from build123d import *

# Parameters (mm, degrees)
SKETCH2_W           = 190
SKETCH2_H           = 90
BOSS_EXTRUDE1_DEPTH = 5
SKETCH3_W           = 190
SKETCH3_H           = 90
SKETCH3_W_2         = 180
SKETCH3_H_2         = 80
BOSS_EXTRUDE2_DEPTH = 25
SKETCH5_W           = 25
SKETCH5_H           = 25
CUT_EXTRUDE1_DEPTH  = 5
SKETCH6_W           = 15
SKETCH6_H           = 15
SKETCH6_R           = 3.25
BOSS_EXTRUDE3_DEPTH = 5
SKETCH8_W           = 184
SKETCH8_H           = 84
CUT_EXTRUDE2_DEPTH  = 27


with BuildPart() as part:
    # Sketch2 → Boss-Extrude1 (new body)
    with BuildSketch(Plane(origin=(0, 0, 0), x_dir=(1, 0, 0), z_dir=(0, 1, 0))):
        Rectangle(SKETCH2_W, SKETCH2_H)
    extrude(amount=BOSS_EXTRUDE1_DEPTH)

    # Sketch3 → Boss-Extrude2 (add)
    with BuildSketch(Plane(origin=(0, 5, 0), x_dir=(1, 0, 0), z_dir=(0, 1, 0))):
        Rectangle(SKETCH3_W, SKETCH3_H)
        Rectangle(SKETCH3_W_2, SKETCH3_H_2, mode=Mode.SUBTRACT)
    extrude(amount=BOSS_EXTRUDE2_DEPTH)

    # Sketch5 → Cut-Extrude1 (cut)
    with BuildSketch(Plane(origin=(-90, 0, 0), x_dir=(0, 0, -1), z_dir=(1, 0, 0))):
        with Locations((-27.5, 17.5)):
            Rectangle(SKETCH5_W, SKETCH5_H)
        with Locations((27.5, 17.5)):
            Rectangle(SKETCH5_W, SKETCH5_H)
    extrude(amount=-CUT_EXTRUDE1_DEPTH, mode=Mode.SUBTRACT)

    # Sketch6 → Boss-Extrude3 (add)
    # profile 1 of 4: a face of its own
    with BuildSketch(Plane(origin=(0, 30, 0), x_dir=(1, 0, 0), z_dir=(0, 1, 0))):
        with Locations((-71.593545043, 52.5)):
            Rectangle(SKETCH6_W, SKETCH6_H)
        with Locations(Location((-71.593545043, 52.5, 0), (0, 0, 270))):
            Circle(SKETCH6_R, mode=Mode.SUBTRACT)
    # profile 2 of 4: a face of its own
    with BuildSketch(Plane(origin=(0, 30, 0), x_dir=(1, 0, 0), z_dir=(0, 1, 0))):
        with Locations((-71.593545043, -52.5)):
            Rectangle(SKETCH6_W, SKETCH6_H)
        with Locations(Location((-71.593545043, -52.5, 0), (0, 0, 90))):
            Circle(SKETCH6_R, mode=Mode.SUBTRACT)
    # profile 3 of 4: a face of its own
    with BuildSketch(Plane(origin=(0, 30, 0), x_dir=(1, 0, 0), z_dir=(0, 1, 0))):
        with Locations((71.593545043, -52.5)):
            Rectangle(SKETCH6_W, SKETCH6_H)
        with Locations(Location((71.593545043, -52.5, 0), (0, 0, 270))):
            Circle(SKETCH6_R, mode=Mode.SUBTRACT)
    # profile 4 of 4: a face of its own
    with BuildSketch(Plane(origin=(0, 30, 0), x_dir=(1, 0, 0), z_dir=(0, 1, 0))):
        with Locations((71.593545043, 52.5)):
            Rectangle(SKETCH6_W, SKETCH6_H)
        with Locations(Location((71.593545043, 52.5, 0), (0, 0, 90))):
            Circle(SKETCH6_R, mode=Mode.SUBTRACT)
    extrude(amount=-BOSS_EXTRUDE3_DEPTH)

    # Sketch8 → Cut-Extrude2 (cut)
    with BuildSketch(Plane(origin=(0, 30, 0), x_dir=(1, 0, 0), z_dir=(0, 1, 0))):
        Rectangle(SKETCH8_W, SKETCH8_H)
    extrude(amount=-CUT_EXTRUDE2_DEPTH, mode=Mode.SUBTRACT)


solid = part.part
Check sheet for the modelled part. Datum: model origin and axes. Units: mm. A direction names the side the tool comes from. Give positions to 0.01 mm unless a question says otherwise; leave off trailing zeros. Loops run counter-clockwise (first coordinate to the right, second up) from the corner with the lowest first, then second, coordinate; pieces in that order, holes last. Notation, with made-up numbers: M 13.5,23 L 50.5,23 A15 cw 50.5,30 Z; hole C 77.25,61 d1. An arc over 180 degrees is marked long. Use a Markdown table: item, result. Add a question column.
Q1. Sectioned sample at D-D, the plane x = 19. Record the cut outline in (y, z).
Q2. Go/stop test with flat-tipped pins: pin 1 (0.9 mm diameter, centred on x = -93.5, y = 19, fed in from +Z); pin 2 (16.5 mm diameter, centred on x = 72.5, z = -55, fed in from -Y); pin 3 (6 mm diameter, centred on x = -35.5, z = -5.5, fed in from +Y); pin 4 (5 mm diameter, centred on x = 71.59, z = 52.5, fed in from +Y). Record where each tip stops, or that it passes through.
Q3. Tool access check on faces 1 (the flat face through (-64.094, 28, 53)), 2 (the flat face through (-64.094, 28, -52)), 3 (the flat face through (79.094, 28, -52)), 4 (the flat face through (-72, 25, -56)). Record the directions out of +Z, -Z, +X, -X, +Y, -Y that give a thin tool (end or side, any length) a straight path to the whole face; none if there is none.
Q4. Sectioned sample at B-B, the plane z = 52.5. Record the cut outline in (x, y).
Q5. Sectioned sample at C-C, the plane z = 11. Record the cut outline in (x, y), then the cut area to 3 significant figures.
Q6. Scan lines: line 1 along X through (y, z) = (27.4, -52.5); line 2 along Z through (x, y) = (-77, 8); line 3 along X through (y, z) = (20.25, 4). Record each from-to range of solid material in increasing order. Write a range as [from, to].
Q7. Sectioned sample at A-A, the plane y = 15. Record the cut outline in (x, z), then the cut area to 3 significant figures.
Verdict:
| question | item | result |
|---|---|---|
| 1 | outline | M 0,-45 L 30,-45 L 30,-42 L 3,-42 L 3,42 L 30,42 L 30,45 L 0,45 Z |
| 2 | pin 1 | z = 45 |
| 2 | pin 2 | y = 25 |
| 2 | pin 3 | y = 3 |
| 2 | pin 4 | through |
| 3 | face 1 | +Z, +Y, -Y |
| 3 | face 2 | -Z, +Y, -Y |
| 3 | face 3 | -Z, +X, +Y, -Y |
| 3 | face 4 | -Z, +X, -X, -Y |
| 4 | outline | M -79.09,25 L -74.84,25 L -74.84,30 L -79.09,30 Z; M -68.34,25 L -64.09,25 L -64.09,30 L -68.34,30 Z; M 64.09,25 L 68.34,25 L 68.34,30 L 64.09,30 Z; M 74.84,25 L 79.09,25 L 79.09,30 L 74.84,30 Z |
| 5 | outline | M -95,0 L 95,0 L 95,30 L 92,30 L 92,3 L -92,3 L -92,30 L -95,30 Z |
| 5 | area | 732 mm^2 |
| 6 | line 1 | [-79.09, -74.84], [-68.34, -64.09], [64.09, 68.34], [74.84, 79.09] |
| 6 | line 2 | [-45, -42], [42, 45] |
| 6 | line 3 | [-95, -92], [92, 95] |
| 7 | outline | M -95,-45 L 95,-45 L 95,45 L -95,45 L -95,40 L -92,40 L -92,42 L 92,42 L 92,-42 L -92,-42 L -92,-40 L -95,-40 Z; M -95,-15 L -92,-15 L -92,15 L -95,15 Z |
| 7 | area | 1,490 mm^2 |
